from build123d import *

# Parameters (mm, degrees)
SKETCH_1_W          = 100
SKETCH_1_H          = 100
SKETCH_1_R          = 1.9
EXTRUDE_1_DEPTH     = 3
SKETCH_2_R          = 38.5
CUT_EXTRUDE_1_DEPTH = 10
SKETCH_3_W          = 100
SKETCH_3_H          = 100
SKETCH_3_W_2        = 94
SKETCH_3_H_2        = 94
EXTRUDE_2_DEPTH     = 60
FILLET_1_R          = 2
CHAMFER_1_SIZE      = 0.4
FILLET_2_R          = 0.8
CHAMFER_2_SIZE      = 0.4
SKETCH_4_W          = 8
SKETCH_4_H          = 12
EXTRUDE_3_DEPTH     = 6
CHAMFER_3_SIZE      = 8
SKETCH_5_R          = 1.4
CUT_EXTRUDE_2_DEPTH = 158.838525082
FILLET_3_R          = 1


with BuildPart() as part:
    # 草图1 → 凸台-拉伸1 (new body)
    with BuildSketch(Plane(origin=(0, 0, 0), x_dir=(1, 0, 0), z_dir=(0, 1, 0))):
        with Locations((50, -50)):
            Rectangle(SKETCH_1_W, SKETCH_1_H)
        with Locations(Location((16.970562748, -83.029437252, 0), (0, 0, 270))):
            Circle(SKETCH_1_R, mode=Mode.SUBTRACT)
        with Locations(Location((87.681240867, -12.318759133, 0), (0, 0, 270))):
            Circle(SKETCH_1_R, mode=Mode.SUBTRACT)
    extrude(amount=EXTRUDE_1_DEPTH)

    # 草图2 → 切除-拉伸1 (cut)
    with BuildSketch(Plane(origin=(0, 3, 0), x_dir=(1, 0, 0), z_dir=(0, 1, 0))):
        with Locations(Location((48.381240867, -50.918759133, 0), (0, 0, 270))):
            Circle(SKETCH_2_R)
    extrude(amount=-CUT_EXTRUDE_1_DEPTH, mode=Mode.SUBTRACT)

    # 草图3 → 凸台-拉伸2 (add)
    with BuildSketch(Plane.XZ):
        with Locations((50, 50)):
            Rectangle(SKETCH_3_W, SKETCH_3_H)
        with Locations((50, 50)):
            Rectangle(SKETCH_3_W_2, SKETCH_3_H_2, mode=Mode.SUBTRACT)
    extrude(amount=EXTRUDE_2_DEPTH)

    # 圆角1
    fillet_1_edges = [part.edges().sort_by_distance(p)[0] for p in [
        (0, -28.5, 0),
        (100, -28.5, 0),
        (100, -28.5, 100),
        (0, -28.5, 100),
    ]]
    fillet(fillet_1_edges, radius=FILLET_1_R)

    # 倒角1
    chamfer_1_edges = [part.edges().sort_by_distance(p)[0] for p in [
        (16.970562748, 3, 81.129437252),
        (87.681240867, 3, 10.418759133),
        (48.381240867, 3, 12.418759133),
        (50, 3, 0),
        (100, 3, 50),
        (0, 3, 50),
        (50, 3, 100),
        (0.585786438, 3, 99.414213562),
        (0.585786438, 3, 0.585786438),
        (99.414213562, 3, 99.414213562),
        (99.414213562, 3, 0.585786438),
    ]]
    chamfer(chamfer_1_edges, length=CHAMFER_1_SIZE)

    # 圆角2
    fillet_2_edges = [part.edges().sort_by_distance(p)[0] for p in [
        (50, 0, 97),
        (3, 0, 50),
        (50, 0, 3),
        (97, 0, 50),
        (3, -30, 97),
        (3, -30, 3),
        (97, -30, 3),
        (97, -30, 97),
    ]]
    fillet(fillet_2_edges, radius=FILLET_2_R)

    # 倒角2
    chamfer_2_edges = [part.edges().sort_by_distance(p)[0] for p in [
        (50, -60, 97),
        (97, -60, 50),
        (50, -60, 3),
        (3, -60, 50),
        (3.234314575, -60, 3.234314575),
        (96.765685425, -60, 3.234314575),
        (96.765685425, -60, 96.765685425),
        (3.234314575, -60, 96.765685425),
        (50, -60, 0),
        (50, -60, 100),
        (0, -60, 50),
        (100, -60, 50),
        (0.585786438, -60, 99.414213562),
        (0.585786438, -60, 0.585786438),
        (99.414213562, -60, 99.414213562),
        (99.414213562, -60, 0.585786438),
    ]]
    chamfer(chamfer_2_edges, length=CHAMFER_2_SIZE)

    # 草图4 → 凸台-拉伸3 (add)
    with BuildSketch(Plane(origin=(0, -54, 0), x_dir=(-1, 0, 0), z_dir=(0, -1, 0))):
        with Locations((-104, -50)):
            Rectangle(SKETCH_4_W, SKETCH_4_H)
        with Locations((4, -50)):
            Rectangle(SKETCH_4_W, SKETCH_4_H)
    extrude(amount=-EXTRUDE_3_DEPTH)

    # 倒角3
    chamfer_3_edges = [part.edges().sort_by_distance(p)[0] for p in [
        (0, -48, 50),
        (100, -48, 50),
    ]]
    chamfer(chamfer_3_edges, length=CHAMFER_3_SIZE - 0.0001)  # a hair under: the kernel refuses the full size

    # 草图5 → 切除-拉伸2 (cut, through all)
    with BuildSketch(Plane(origin=(0, -54, 0), x_dir=(-1, 0, 0), z_dir=(0, -1, 0))):
        with Locations(Location((5, -50, 0), (0, 0, 90))):
            Circle(SKETCH_5_R)
        with Locations(Location((-105, -50, 0), (0, 0, 90))):
            Circle(SKETCH_5_R)
    extrude(amount=-CUT_EXTRUDE_2_DEPTH, mode=Mode.SUBTRACT)

    # 圆角3
    fillet_3_edges = [part.edges().sort_by_distance(p)[0] for p in [
        (100, -47.00005, 44),
        (100, -47.00005, 56),
        (108, -51, 56),
        (108, -51, 44),
        (0, -47.00005, 56),
        (0, -47.00005, 44),
        (-8, -51, 44),
        (-8, -51, 56),
    ]]
    fillet(fillet_3_edges, radius=FILLET_3_R)


solid = part.part
The listing builds one solid part. Answer for the finished solid, in the listing's coordinates (mm). A direction names the side the tool comes from. Coordinates: 2 decimals unless noted, no trailing zeros. Write each loop counter-clockwise with the first axis right and the second up, starting at its lowest first coordinate (ties: lowest second). Pieces come first, ordered by that corner, then holes. Notation, with made-up numbers: (-10.75, -24.5) - (22.25, -24.5) arc R15 cw to (22.25, -11.5) - close; hole circle Ø5 at (37.5, 30.5). An arc over 180 degrees is marked (long way). Put each result on its own line as item: value.
1. The part is cut by section B-B on y = -52. State how many separate pieces and enclosed holes the cut face has, plus the area to 3 significant figures.
Answer sheet:
separate pieces: 1
enclosed holes: 3
area: 1,340 mm^2
2. A tool of negligible diameter and unlimited length cuts with its end or side. For faces 4 (the face through (80.2, 0, 28.8)), 5 (the face through (-4, -49, 44)), 6 (the face through (-3, -54, 50)), from which of +Z, -Z, +X, -X, +Y, -Y can it reach the whole face along a straight path? Write none if from no direction.
Answer sheet:
face 4: -Y
face 5: -Z, -X, +Y, -Y
face 6: +Z, -Z, -X, -Y
3. Flat-ended cylindrical pins translate along their axes: pin 1 Ø5 at (x, y) = (-4, -46.5) entering from +Z; pin 2 Ø18.5 at (y, z) = (-20.5, 27) entering from +X; pin 3 Ø10 at (y, z) = (-6, 56.5) entering from -X; pin 4 Ø2.5 at (x, z) = (87.68, 12.32) entering from +Y (3 decimals). Find the tip coordinate at first contact, or state that the pin passes through.
Answer sheet:
pin 1: stops at z = 56
pin 2: stops at x = 100
pin 3: stops at x = 0
pin 4: passes through
4. Determine the mould class of faces 1 (the face through (-3, -43, 50)), 2 (the face through (17.541, 1.282, 84.842)), 3 (the face through (-4, -49, 56)) for opening direction Z: pulls with the +Z half, pulls with the -Z half, needs draft (parallel to the pull), parting line crosses it, or undercut.
Answer sheet:
face 1: needs draft
face 2: undercut
face 3: pulls with the +Z half
5. The part is cut by section A-A on y = -25. Give the vertices of the cut face in (x, z).
Answer sheet:
outline: (0, 2) arc R2 ccw to (2, 0) - (98, 0) arc R2 ccw to (100, 2) - (100, 98) arc R2 ccw to (98, 100) - (2, 100) arc R2 ccw to (0, 98) - close; hole (3, 3.8) arc R0.8 ccw to (3.8, 3) - (96.2, 3) arc R0.8 ccw to (97, 3.8) - (97, 96.2) arc R0.8 ccw to (96.2, 97) - (3.8, 97) arc R0.8 ccw to (3, 96.2) - close
6. The part is cut by section C-C on x = -5. Give the vertices of the cut face in (y, z), plus the area to 3 significant figures.
Answer sheet:
outline: (-54, 44) - (-45, 44) - (-45, 48.6) - (-54, 48.6) - close; (-54, 51.4) - (-45, 51.4) - (-45, 56) - (-54, 56) - close
area: 82.8 mm^2
7. Find the intervals of material crossed by line 1 along X through (y, z) = (-49.75, 50); line 2 along X through (y, z) = (-38.5, 55); line 3 along Z through (x, y) = (-5, -50.5), in increasing order. Write a range as from..to.
Answer sheet:
line 1: x = -8..-6.4, -3.6..3, 97..103.6, 106.4..108
line 2: x = 0..3, 97..100
line 3: z = 44..48.6, 51.4..56
